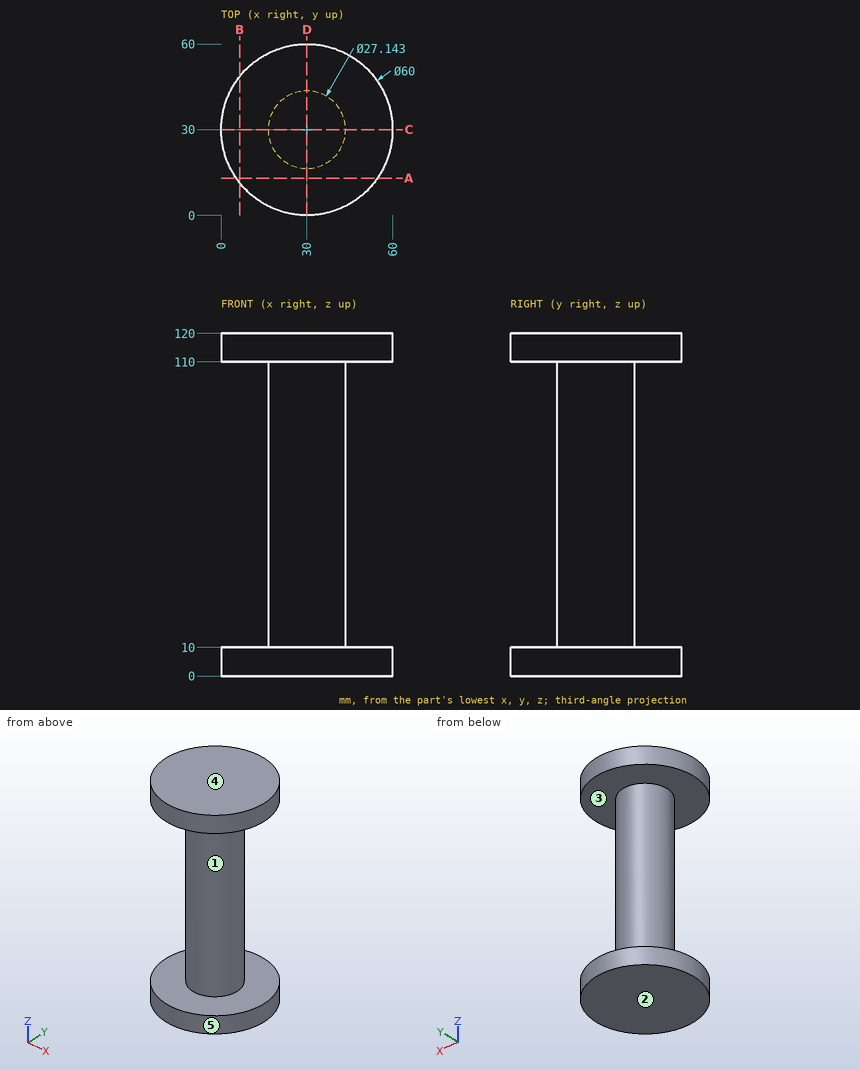
Input: dimensioned drawing with shaded views. Units: mm. Origin: part minimum x, y, z. A direction names the side the tool comes from. Round coordinates to 2 decimals unless told otherwise and drop trailing zeros. Order: outer loops, then holes, each group sorted by start corner. A loop starts at its lowest first (then second) coordinate and runs counter-clockwise, first axis right, second up. Notation, with made-up numbers: (-23, 32) - (28, 32) arc R25 ccw to (28, 62) - close; hole circle Ø2 at (-4.75, 63). An arc over 180 degrees is marked (long way). Write item = value, one per line. Start each with the question number.
Q1. Cut plane A-A on y = 13. Return the cut outline in (x, z).
Q2. Pin query (flat end, axial travel): pin 1 (8 mm diameter, centred on y = 27, z = 60, fed in from -X); pin 2 (12 mm diameter, centred on y = 23, z = 87, fed in from -X); pin 3 (8 mm diameter, centred on y = 18, z = 40, fed in from -X). Return the tip coordinate at first contact, or that it passes through.
Q3. Cut plane C-C on y = 30. Return the cut outline in (x, z).
Q4. Cut plane B-B on x = 6.5. Return the cut outline in (y, z).
Q5. Ray query, line 1 (Z direction, x = 50.5, y = 25.5); line 2 (Y direction, x = 30.5, z = 50); line 3 (X direction, y = 30.5, z = 8). Return the intervals inside material, ascending. Write a range as from..to.
Q6. Pull-direction query (Z, two-part tool) for the marked faces 3, 4 and 5; classes: +Z half, -Z half, draft (parallel to the pull), parting line (faces both ways), or undercut.
Q7. Access query for the marked faces 1 and 2. Directions: +Z, -Z, +X, -X, +Y, -Y. A direction counts if a zero-diameter tool reaches every point of the face in a straight line with its end or side. Return the directions, or none.
Outcome:
q1.outline = (5.28, 0) - (54.72, 0) - (54.72, 10) - (5.28, 10) - close; (5.28, 110) - (54.72, 110) - (54.72, 120) - (5.28, 120) - close
q2.pin_1 = 16.43
q2.pin_2 = 16.47
q2.pin_3 = 19.04
q3.outline = (0, 0) - (60, 0) - (60, 10) - (43.57, 10) - (43.57, 110) - (60, 110) - (60, 120) - (0, 120) - (0, 110) - (16.43, 110) - (16.43, 10) - (0, 10) - close
q4.outline = (11.35, 0) - (48.65, 0) - (48.65, 10) - (11.35, 10) - close; (11.35, 110) - (48.65, 110) - (48.65, 120) - (11.35, 120) - close
q5.line_1 = 0..10, 110..120
q5.line_2 = 16.44..43.56
q5.line_3 = 0..60
q6.face_3 = undercut
q6.face_4 = +Z half
q6.face_5 = draft
q7.face_1 = none
q7.face_2 = -Z, +X, -X, +Y, -Y
